from build123d import *

# Parameters (mm, degrees)
F0_W     = 30
F0_H     = 41.5
F1_DEPTH = 2
F2_W     = 20
F2_H     = 31
F3_DEPTH = 5
F4_W     = 16.5
F4_H     = 20.7
F5_DEPTH = 25
F6_R     = 2


with BuildPart() as f1:
    # F0 (on Top) → F1 (new body)
    with BuildSketch(Plane.XY):
        with Locations((0.211424, -1.432606)):
            Rectangle(F0_W, F0_H)
    extrude(amount=F1_DEPTH)

    # F2 (on face) → F3 (join)
    with BuildSketch(Plane(origin=(0, 0, 0), x_dir=(1, 0, 0), z_dir=(0, 0, -1))):
        with Locations((0.211424, 1.682606)):
            Rectangle(F2_W, F2_H)
    extrude(amount=F3_DEPTH)

    # F4 (on face) → F5 (cut)
    with BuildSketch(Plane(origin=(0, 0, -5), x_dir=(1, 0, 0), z_dir=(0, 0, -1))):
        with Locations((0.211424, 4.832606)):
            Rectangle(F4_W, F4_H)
    extrude(amount=-F5_DEPTH, mode=Mode.SUBTRACT)

    # F6
    f6_edges = [f1.edges().sort_by_distance(p)[0] for p in [
        (8.461424, -4.832606, 2),
        (0.211424, 5.517394, 2),
        (-8.038576, -4.832606, 2),
        (0.211424, -15.182606, 2),
    ]]
    fillet(f6_edges, radius=F6_R)


solid = f1.part
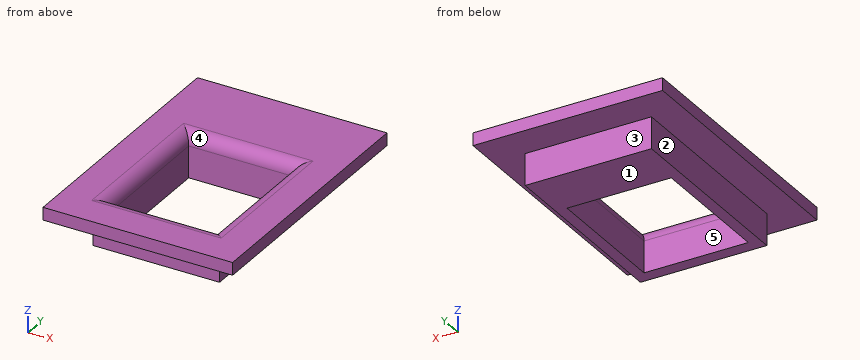
Source: CAD feature listing. Evaluate the final solid. Frame: model axes, mm. Face numbers are marked on the shaded views. A direction names the side the tool comes from. Coordinates: 2 decimals unless noted, no trailing zeros. Loops run counter-clockwise (first coordinate to the right, second up) from the corner with the lowest first, then second, coordinate; pieces in that order, holes last. Notation, with made-up numbers: (-12.75, 18.25) - (8.25, 18.25) arc R13 ccw to (8.25, 23.25) - close; hole circle Ø7 at (56, -37.75). An arc over 180 degrees is marked (long way). One line per item, written item: value. Start each with the question number.
1. Set-up query: the marked faces 1, 2, 3, 4 and 5. Return all of +Z, -Z, +X, -X, +Y, -Y with unobstructed straight access to the full face (end or side cutting, diameter ignored); none if empty.
2. Section B-B (z = -2.5). Return the cut outline in (x, y), and give its area (3 significant figures).
3. Section A-A (x = 2.5). Return the cut outline in (y, z), and give its area (3 significant figures).
4. Section C-C (y = -14). Return the cut outline in (x, z), and give its area (3 significant figures).
5. Contact query for flat-ended pins moving along their axis: P1, Ø2.5, axis at y = -0.5, z = -2.5, coming from the -X side; P2, Ø2.5, axis at y = -5, z = -2, coming from the +X side; P3, Ø2.5, axis at x = 1, z = -3.5, coming from the -Y side. Output: stop coordinate, or through.
6. Section D-D (y = 12). Return the cut outline in (x, z), and give its area (3 significant figures).
7. Ray query, L1, parallel to Y at x = -1, z = -3.25; L2, parallel to X at y = 4.5, z = -2.25; L3, parallel to Z at x = -10, y = 6.5. Return the intervals inside material, ascending.
Verdict:
1. face 1: -Z, +X, -X, +Y, -Y
1. face 2: -Z, -X, +Y, -Y
1. face 3: -Z, +X, -X, +Y
1. face 4: +Z
1. face 5: +Z, -Z
2. outline: (-9.79, -17.18) - (10.21, -17.18) - (10.21, 13.82) - (-9.79, 13.82) - close; hole (-8.04, -15.18) - (8.46, -15.18) - (8.46, 5.52) - (-8.04, 5.52) - close
2. area: 278 mm2
3. outline: (-22.18, 0) - (-17.18, 0) - (-17.18, -5) - (-15.18, -5) - (-15.18, 0) arc R2 ccw to (-17.18, 2) - (-22.18, 2) - close; (5.52, -5) - (13.82, -5) - (13.82, 0) - (19.32, 0) - (19.32, 2) - (7.52, 2) arc R2 ccw to (5.52, 0) - close
3. area: 91.4 mm2
4. outline: (-14.79, 0) - (-9.79, 0) - (-9.79, -5) - (-8.04, -5) - (-8.04, 0) arc R2 ccw to (-10.04, 2) - (-14.79, 2) - close; (8.46, -5) - (10.21, -5) - (10.21, 0) - (15.21, 0) - (15.21, 2) - (10.46, 2) arc R2 ccw to (8.46, 0) - close
4. area: 42.8 mm2
5. P1: stops at x = -9.79
5. P2: stops at x = 10.21
5. P3: stops at y = -17.18
6. outline: (-14.79, 0) - (-9.79, 0) - (-9.79, -5) - (10.21, -5) - (10.21, 0) - (15.21, 0) - (15.21, 2) - (-14.79, 2) - close
6. area: 160 mm2
7. L1: y = -17.18 to -15.18, 5.52 to 13.82
7. L2: x = -9.79 to -8.04, 8.46 to 10.21
7. L3: z = 0 to 2
